```python
from build123d import *

# Parameters (mm, degrees)
BOSS_EXTRUDE1_DEPTH         = 13.352390271
SKETCH4_R                   = 38.89375
BOSS_EXTRUDE2_DEPTH         = 4.7625
CUT_EXTRUDE1_DEPTH          = 91.22895136
CUT_EXTRUDE1_DEPTH_BACK     = 91.22895136
SKETCH2_R                   = 6.35
SKETCH5_R                   = 38.89375
SKETCH5_R_2                 = 28.575
BOSS_EXTRUDE3_DEPTH         = 1.5875
F_1_4_20_TAPPED_HOLE1_D     = 5.1054
F_1_4_20_TAPPED_HOLE2_D     = 5.1054
F_1_4_20_TAPPED_HOLE2_DEPTH = 118.27002
F_1_4_20_TAPPED_HOLE2_TIP   = 1.533816902


with BuildPart() as part:
    # Sketch1 → Boss-Extrude1 (new body)
    with BuildSketch(Plane(origin=(0, 0, 0), x_dir=(1, 0, 0), z_dir=(0, 1, 0))):
        with BuildLine():
            Line((-15.875, 0), (-15.875, 79.375))
            Line((-15.875, 79.375), (15.875, 79.375))
            Line((15.875, 79.375), (15.875, 0))
            ThreePointArc((15.875, 0), (0, -15.875), (-15.875, 0))
        make_face()
    extrude(amount=BOSS_EXTRUDE1_DEPTH)

    # Sketch4 → Boss-Extrude2 (add)
    with BuildSketch(Plane.XZ):
        with Locations(Location((0, 0, 0), (0, 0, 245.910493888))):
            Circle(SKETCH4_R)
    extrude(amount=BOSS_EXTRUDE2_DEPTH)

    # Sketch2 → Cut-Extrude1 (cut, two sides: drawn at the far end of the back side and taken through both)
    with BuildSketch(Plane(origin=(0, 13.352390271, 0), x_dir=(1, 0, 0), z_dir=(0, 1, 0)).offset(-CUT_EXTRUDE1_DEPTH_BACK)):
        with Locations(Location((0, 0, 0), (0, 0, 270))):
            Circle(SKETCH2_R)
    extrude(amount=CUT_EXTRUDE1_DEPTH + CUT_EXTRUDE1_DEPTH_BACK, mode=Mode.SUBTRACT)

    # Sketch5 → Boss-Extrude3 (add)
    with BuildSketch(Plane.XZ.offset(4.7625)):
        with Locations(Location((0, 0, 0), (0, 0, 245.910493888))):
            Circle(SKETCH5_R)
        with Locations(Location((0, 0, 0), (0, 0, 270))):
            Circle(SKETCH5_R_2, mode=Mode.SUBTRACT)
    extrude(amount=BOSS_EXTRUDE3_DEPTH)

    # 1/4-20 Tapped Hole1 (through all)
    with Locations(Plane(origin=(0, 0, -79.375), x_dir=(-1, 0, 0), z_dir=(0, 0, -1))):
        with Locations((0, 6.676195135)):
            Hole(F_1_4_20_TAPPED_HOLE1_D / 2)

    # 1/4-20 Tapped Hole2
    with Locations(Plane(origin=(0, 13.352390271, 0), x_dir=(1, 0, 0), z_dir=(0, 1, 0))):
        with Locations((-9.525, 69.85), (9.525, 69.85), (0, 11.1125)):
            Hole(F_1_4_20_TAPPED_HOLE2_D / 2, depth=F_1_4_20_TAPPED_HOLE2_DEPTH)
            with Locations((0, 0, -(F_1_4_20_TAPPED_HOLE2_DEPTH + F_1_4_20_TAPPED_HOLE2_TIP / 2))):  # 118° drill point
                Cone(0, F_1_4_20_TAPPED_HOLE2_D / 2, F_1_4_20_TAPPED_HOLE2_TIP, mode=Mode.SUBTRACT)


solid = part.part
```
Geometry: final body of the model. Coordinates: model frame, mm. A direction names the side the tool comes from. Round coordinates to 2 decimals unless told otherwise and drop trailing zeros. Loops run counter-clockwise (first coordinate to the right, second up) from the corner with the lowest first, then second, coordinate; pieces in that order, holes last. Notation, with made-up numbers: (-9.75, -27.5) -> (0.25, -27.5) arc R24 cw to (0.25, -10.5) -> close; hole circle Ø1 at (55, -23). An arc over 180 degrees is marked (long way). Use one line per item in the form item = value. Start each with the question number.
1) Section B-B on y = 5.5. Give the number of separate pieces and of enclosed holes in the cut face, then the cut area to 3 significant figures.
2) Line query: L1, parallel to X at y = -5.9, z = 0 (3 decimals); L2, parallel to X at y = 7, z = -63.5 (3 decimals); L3, parallel to X at y = 3.25, z = -69.85 (3 decimals). Output: solid intervals per line, ascending.
3) Section A-A on z = -69.85. Output: boundary loops of the cut face in (x, y) (3 decimals), then the cut area to 3 significant figures.
4) Section D-D on z = -44.5. Output: boundary loops of the cut face in (x, y) (3 decimals), then the cut area to 3 significant figures.
5) First-contact query: P1, Ø4, axis at y = 6, z = -4.5, coming from the +X side (3 decimals); P2, Ø5, axis at y = 11.5, z = 7, coming from the +X side; P3, Ø8, axis at x = 0, z = -11.11, coming from the -Y side; P4, Ø6, axis at x = 0, y = 6.68, coming from the -Z side (3 decimals). Flat tips, straight axial feed; report the tip coordinate or a pass-through.
6) Draft query along X for faces 1 (the cylindrical face through (-0.332, 9.207, 10.916)), 2 (the flat face through (0, 0, -58)), 3 (the flat face through (-15.875, 7, -39)), 4 (the cylindrical face through (2.55, -0.39, -11.22)). Return one class per face: released by +X, released by -X, zero draft, split by the parting line, or undercut.
7) Access query for faces 5 (the flat face through (8, 0, 16)), 6 (the cylindrical face through (1.256, -5.545, 28.547)), 7 (the cylindrical face through (-2.55, 6.79, -7.84)), 8 (the flat face through (15.875, 7, -40)). Directions: +Z, -Z, +X, -X, +Y, -Y. A direction counts if a zero-diameter tool reaches every point of the face in a straight line with its end or side. Return the directions, or none.
Response:
q1.separate_pieces = 2
q1.enclosed_holes = 2
q1.area = 2,370 mm^2
q2.L1 = -38.894 to -28.575, 28.575 to 38.894
q2.L2 = -15.875 to -2.532, 2.532 to 15.875
q2.L3 = -15.875 to -12.078, -6.972 to 6.972, 12.078 to 15.875
q3.outline = (-15.875, 0) -> (-12.078, 0) -> (-12.078, 13.352) -> (-15.875, 13.352) -> close; (-6.972, 0) -> (6.972, 0) -> (6.972, 13.352) -> (-6.972, 13.352) -> close; (12.078, 0) -> (15.875, 0) -> (15.875, 13.352) -> (12.078, 13.352) -> close; hole circle Ø5.105 at (0, 6.676)
q3.area = 267 mm^2
q4.outline = (-15.875, 0) -> (15.875, 0) -> (15.875, 13.352) -> (-15.875, 13.352) -> close; hole circle Ø5.105 at (0, 6.676)
q4.area = 403 mm^2
q5.P1 = 15.875
q5.P2 = 15.22
q5.P3 = -4.76
q5.P4 = -79.375
q6.face_1 = undercut
q6.face_2 = zero draft
q6.face_3 = released by -X
q6.face_4 = undercut
q7.face_5 = +Z, +Y
q7.face_6 = -Y
q7.face_7 = +Z, -Z
q7.face_8 = +Z, -Z, +X, +Y
